```python
from build123d import *

# Parameters (mm, degrees)
F1_DEPTH = 6
F2_R     = 10
F3_R     = 10
F4_R     = 10
F5_R     = 4
F6_R     = 4
F7_R     = 5.08
F8_R     = 5.08


with BuildPart() as f1:
    # F0 (on Right) → F1 (new body)
    with BuildSketch(Plane.YZ):
        with BuildLine():
            Line((206.182857, -370.988358), (206.182857, 379.011642))
            Line((206.182857, 379.011642), (-115.060672, 379.011642))
            Line((-115.060672, 379.011642), (-164.283467, 187.301795))
            ThreePointArc((-164.283467, 187.301795), (-34.827874, 10.767053), (40.379739, -194.82254))
            Line((40.379739, -194.82254), (-41.226477, -227.205956))
            Line((-41.226477, -227.205956), (11.882335, -370.988358))
            Line((11.882335, -370.988358), (206.182857, -370.988358))
        make_face()
    extrude(amount=F1_DEPTH)

    # F2
    f2_edges = [f1.edges().sort_by_distance(p)[0] for p in [
        (3, -41.226477, -227.205956),
    ]]
    fillet(f2_edges, radius=F2_R)

    # F3
    f3_edges = [f1.edges().sort_by_distance(p)[0] for p in [
        (3, 40.379739, -194.82254),
    ]]
    fillet(f3_edges, radius=F3_R)

    # F4
    f4_edges = [f1.edges().sort_by_distance(p)[0] for p in [
        (3, 11.882335, -370.988358),
    ]]
    fillet(f4_edges, radius=F4_R)

    # F5
    f5_edges = [f1.edges().sort_by_distance(p)[0] for p in [
        (3, 206.182857, -370.988358),
    ]]
    fillet(f5_edges, radius=F5_R)

    # F6
    f6_edges = [f1.edges().sort_by_distance(p)[0] for p in [
        (3, 206.182857, 379.011642),
    ]]
    fillet(f6_edges, radius=F6_R)

    # F7
    f7_edges = [f1.edges().sort_by_distance(p)[0] for p in [
        (3, -164.283467, 187.301795),
    ]]
    fillet(f7_edges, radius=F7_R)

    # F8
    f8_edges = [f1.edges().sort_by_distance(p)[0] for p in [
        (3, -115.060672, 379.011642),
    ]]
    fillet(f8_edges, radius=F8_R)


solid = f1.part
```
Could you check a few things on this model? Use its own coordinates, in mm. A direction names the side the tool comes from. Coordinates: 2 decimals unless noted, no trailing zeros. Order: outer loops, then holes, each group sorted by start corner. A loop starts at its lowest first (then second) coordinate and runs counter-clockwise, first axis right, second up. Notation, with made-up numbers: M 11,-11 L 70,-11 A19 cw 70,24 Z; hole C 28.5,-36.75 d2. An arc over 180 degrees is marked long. Use a Markdown table: item, result. Add a question column.
Q1. I want a section at B-B on x = 1.3. List the corners of the cut face in (y, z) for me, then the cut area to 3 significant figures.
Q2. Which directions (+Z, -Z, +X, -X, +Y, -Y) give clear straight access to the entire face, cutting with the end or side of a thin tool? Please do faces 1 (the flat face through (0, 60, 93)), 2 (the cylindrical face through (3, -37.6, 15.9)).
Q3. I want a section at C-C on z = -90. List the corners of the cut face in (x, y) for me, then the cut area to 3 significant figures.
Q4. If I drill on L1, parallel to Y at x = 2.8, z = 142.5; L2, parallel to Y at x = 4.85, z = -196.5; L3, parallel to Z at x = 2.7, y = -77, over which ranges is the centre line in solid material (lowest first)?
Q5. I want a section at A-A on y = -22. List the corners of the cut face in (x, z) for me, then the cut area to 3 significant figures.
Q6. I want a section at D-D on y = -95.5. List the corners of the cut face in (x, z) for me.
Checked values:
| question | item | result |
|---|---|---|
| 1 | outline | M -163.57,190.06 A5.08 ccw -162.3,185.26 A778.75 cw 38.55,-186.47 A10 cw 32.49,-197.96 L -32.15,-223.6 A10 ccw -37.84,-236.36 L 9.47,-364.45 A10 ccw 18.85,-370.99 L 202.18,-370.99 A4 ccw 206.18,-366.99 L 206.18,375.01 A4 ccw 202.18,379.01 L -111.12,379.01 A5.08 ccw -116.04,375.19 Z |
| 1 | area | 198,000 mm² |
| 2 | face 1 | +Z, -Z, -X, +Y, -Y |
| 2 | face 2 | +X, -X, -Y |
| 3 | outline | M 0,10.27 L 6,10.27 L 6,206.18 L 0,206.18 Z |
| 3 | area | 1,180 mm² |
| 4 | L1 | -123.79 to 206.18 |
| 4 | L2 | 35.01 to 206.18 |
| 4 | L3 | 80.48 to 379.01 |
| 5 | outline | M 0,-279.26 L 6,-279.26 L 6,-219.58 L 0,-219.58 Z; M 0,-14.26 L 6,-14.26 L 6,379.01 L 0,379.01 Z |
| 5 | area | 2,720 mm² |
| 6 | outline | M 0,106.56 L 6,106.56 L 6,379.01 L 0,379.01 Z |
